Geometry: final body of the model. Coordinates: model frame, mm. A direction names the side the tool comes from. Give positions to 0.01 mm unless a question says otherwise; leave off trailing zeros. Write each loop counter-clockwise with the first axis right and the second up, starting at its lowest first coordinate (ties: lowest second). Pieces come first, ordered by that corner, then holes. Notation, with made-up numbers: M -36,19.5 L 6,19.5 A29 ccw 6,52.5 Z; hole C 69.25,77.25 d10. An arc over 180 degrees is marked long. Use one line per item in the form item = value. Start each with the question number.
Item 1: Access query for faces 3 (the cylindrical face through (8.584, 2.703, 8.028)), 4 (the flat face through (-10, 2.5, 9)), 5 (the cylindrical face through (7.678, 2.418, 2.958)), 6 (the flat face through (7, -7, 10)), 7 (the flat face through (0, 10, 7)). Directions: +Z, -Z, +X, -X, +Y, -Y. A direction counts if a zero-diameter tool reaches every point of the face in a straight line with its end or side. Return the directions, or none.
Item 2: Section query A-A on y = 0. Return loops of the section in (x, z).
Item 3: Section query C-C on z = 9.25. Return loops of the section in (x, y).
Item 4: Pull-direction query (Y, two-part tool) for faces 1 (the flat face through (2.5, 10, 9)), 2 (the flat face through (10, 2.5, 9)); classes: released by +Y, released by -Y, zero draft, split by the parting line, or undercut.
Item 5: Section query D-D on y = 10.25. Return loops of the section in (x, z), then the cut area to 3 significant figures.
Item 6: Material intervals for line 1 along Y through (x, z) = (0, 2.1); line 2 along X through (y, z) = (-0.75, 2.5); line 3 along X through (y, z) = (-4.75, 0.75), sorted ascending. Write a range as from..to.
Item 7: Contact query for flat-ended pins moving along their axis: P1, Ø1.7, axis at x = 11, y = 0.5, coming from the +Z side; P2, Ø0.9, axis at x = -9.5, z = 9, coming from the +Y side; P3, Ø3, axis at x = -8.5, z = 7.5, coming from the -Y side; P4, Ø2, axis at x = 5.5, y = 1.5, coming from the -Z side. Output: stop coordinate, or through.
from build123d import *

# Parameters (mm, degrees)
SKETCH_1_R          = 12
SKETCH_1_R_2        = 8.05
EXTRUDE_1_DEPTH     = 10
CUT_EXTRUDE_1_DEPTH = 3
SKETCH_4_R          = 9
CUT_EXTRUDE_2_DEPTH = 4


with BuildPart() as part:
    # 草图1 → 凸台-拉伸1 (new body)
    with BuildSketch(Plane.XY):
        Circle(SKETCH_1_R)
        Circle(SKETCH_1_R_2, mode=Mode.SUBTRACT)
    extrude(amount=EXTRUDE_1_DEPTH)

    # 草图3 → 切除-拉伸1 (cut)
    with BuildSketch(Plane.XY.offset(10)):
        Polygon((-16.5, 2.5), (-2.5, 2.5), (-2.5, 16.5), (2.5, 16.5), (2.5, 2.5), (16.5, 2.5), (16.5, -2.5), (2.5, -2.5), (2.5, -16.5), (-2.5, -16.5), (-2.5, -2.5), (-16.5, -2.5), align=None)
    extrude(amount=-CUT_EXTRUDE_1_DEPTH, mode=Mode.SUBTRACT)

    # 草图4 → 切除-拉伸2 (cut)
    with BuildSketch(Plane.XY.offset(10)):
        Circle(SKETCH_4_R)
    extrude(amount=-CUT_EXTRUDE_2_DEPTH, mode=Mode.SUBTRACT)


solid = part.part
Answer sheet:
q1.face_3 = +Z
q1.face_4 = +Z, +X, -X
q1.face_5 = +Z, -Z
q1.face_6 = +Z, +X, -X, +Y, -Y
q1.face_7 = +Z, +Y, -Y
q2.outline = M -12,0 L -8.05,0 L -8.05,6 L -9,6 L -9,7 L -12,7 Z; M 8.05,0 L 12,0 L 12,7 L 9,7 L 9,6 L 8.05,6 Z
q3.outline = M -11.74,-2.5 A12 ccw -2.5,-11.74 L -2.5,-8.65 A9 cw -8.65,-2.5 Z; M -11.74,2.5 L -8.65,2.5 A9 cw -2.5,8.65 L -2.5,11.74 A12 ccw Z; M 2.5,-11.74 A12 ccw 11.74,-2.5 L 8.65,-2.5 A9 cw 2.5,-8.65 Z; M 2.5,8.65 A9 cw 8.65,2.5 L 11.74,2.5 A12 ccw 2.5,11.74 Z
q4.face_1 = zero draft
q4.face_2 = undercut
q5.outline = M -6.24,0 L 6.24,0 L 6.24,10 L 2.5,10 L 2.5,7 L -2.5,7 L -2.5,10 L -6.24,10 Z
q5.area = 110 mm2
q6.line_1 = -12..-8.05, 8.05..12
q6.line_2 = -11.98..-8.01, 8.01..11.98
q6.line_3 = -11.02..-6.5, 6.5..11.02
q7.P1 = 7
q7.P2 = 7.88
q7.P3 = -9.75
q7.P4 = through
